For this review, use the dimensioned drawing (mm, ordinates from the lowest corner) and the shaded views. A direction names the side the tool comes from. Coordinates: 2 decimals unless noted, no trailing zeros. Loops run counter-clockwise (first coordinate to the right, second up) from the corner with the lowest first, then second, coordinate; pieces in that order, holes last. Notation, with made-up numbers: (47.5, 6.25) - (97.5, 6.25) arc R19 cw to (97.5, 22.25) - close; hole circle Ø1 at (56, -14). An arc over 180 degrees is marked (long way). Use a Markdown table: item, result. Add a question column.
1) Add section B-B, the plane x = 63.5. Give the boundary of the cut face in (y, z) (1 decimal), and give its area (3 significant figures).
2) For the marked faces 1, 2 and 3, list the 3-axis set-ups (+Z, -Z, +X, -X, +Y, -Y) from which the entire face can be reached by the end or side of a thin tool; tool diameter is ignored.
3) To check wall thickness, follow L1, parallel to Y at x = 74, z = 14; L2, parallel to X at y = 25.5, z = 7.5 (1 decimal); L3, parallel to X at y = 25, z = 6 (1 decimal). State the ranges of each line that lie inside material, in increasing order. Write a range as [from, to].
4) Add section A-A, the plane y = 25.4. Give the number of separate pieces and of enclosed holes in the cut face.
5) Clearance check with flat-ended pins moving along their axes: pin 1 (5 mm diameter, centred on y = 41, z = 3, fed in from -X); pin 2 (8 mm diameter, centred on x = 41.275, y = 76.2, fed in from -Z) (1 decimal); pin 3 (4 mm diameter, centred on y = 112.5, z = 15.5, fed in from -X); pin 4 (5.5 mm diameter, centred on y = 3, z = 23, fed in from +X). State where each tip first meets the part, or that it passes through.
6) The part is to be moulded in two halves that separate along Y. For the marked faces 4, 5 and 6, say which applies: pulls with the +Y half, pulls with the -Y half, needs draft (parallel to the pull), parting line crosses it, or undercut.
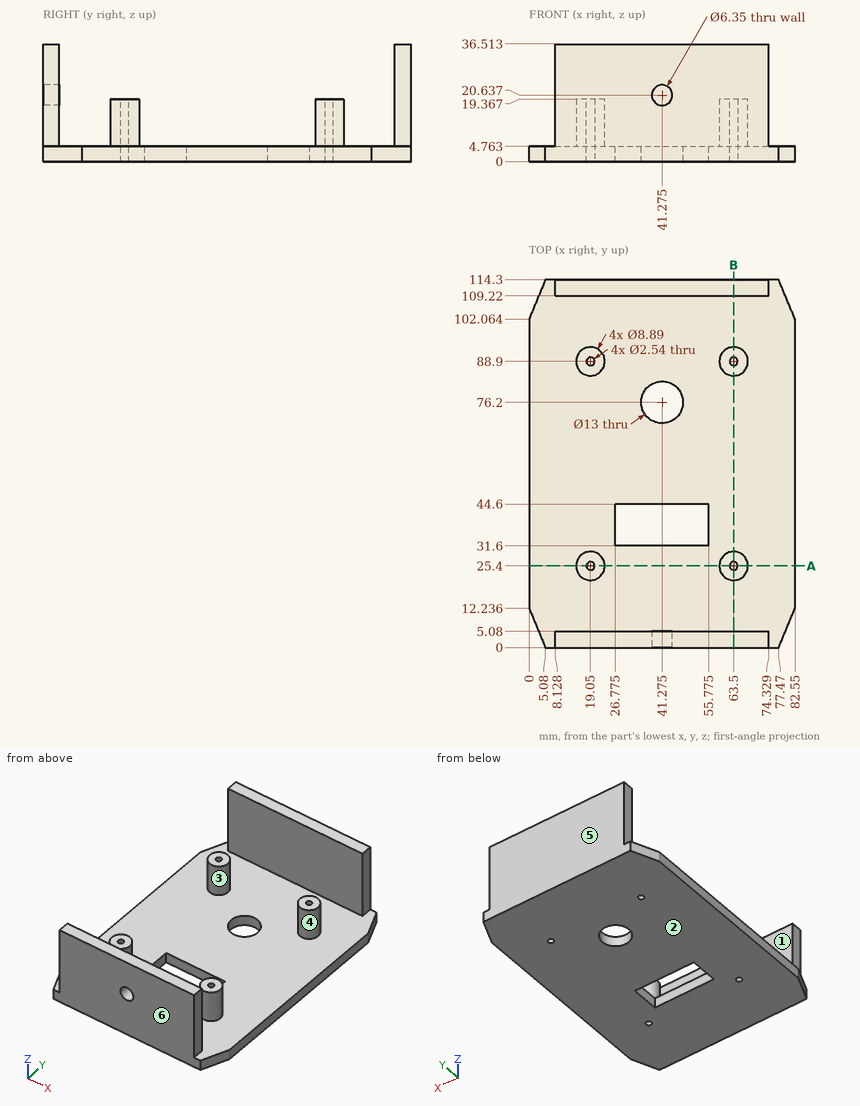
From the geometry:
| question | item | result |
|---|---|---|
| 1 | outline | (0, 0) - (24.1, 0) - (24.1, 19.4) - (21, 19.4) - (21, 4.8) - (5.1, 4.8) - (5.1, 36.5) - (0, 36.5) - close; (26.7, 0) - (87.6, 0) - (87.6, 19.4) - (84.5, 19.4) - (84.5, 4.8) - (29.8, 4.8) - (29.8, 19.4) - (26.7, 19.4) - close; (90.2, 0) - (114.3, 0) - (114.3, 36.5) - (109.2, 36.5) - (109.2, 4.8) - (93.3, 4.8) - (93.3, 19.4) - (90.2, 19.4) - close |
| 1 | area | 1,030 mm^2 |
| 2 | face 1 | +Z, +X, -X |
| 2 | face 2 | -Z, +X, -X, +Y, -Y |
| 2 | face 3 | +Z |
| 3 | L1 | y = [0, 5.08], [109.22, 114.3] |
| 3 | L2 | x = [14.6, 17.8], [20.3, 23.5], [59.1, 62.2], [64.8, 67.9] |
| 3 | L3 | x = [14.6, 17.8], [20.3, 23.5], [59.1, 62.3], [64.7, 67.9] |
| 4 | separate pieces | 3 |
| 4 | enclosed holes | 0 |
| 5 | pin 1 | stops at x = 0 |
| 5 | pin 2 | passes through |
| 5 | pin 3 | stops at x = 8.13 |
| 5 | pin 4 | stops at x = 74.33 |
| 6 | face 4 | undercut |
| 6 | face 5 | pulls with the +Y half |
| 6 | face 6 | pulls with the -Y half |
